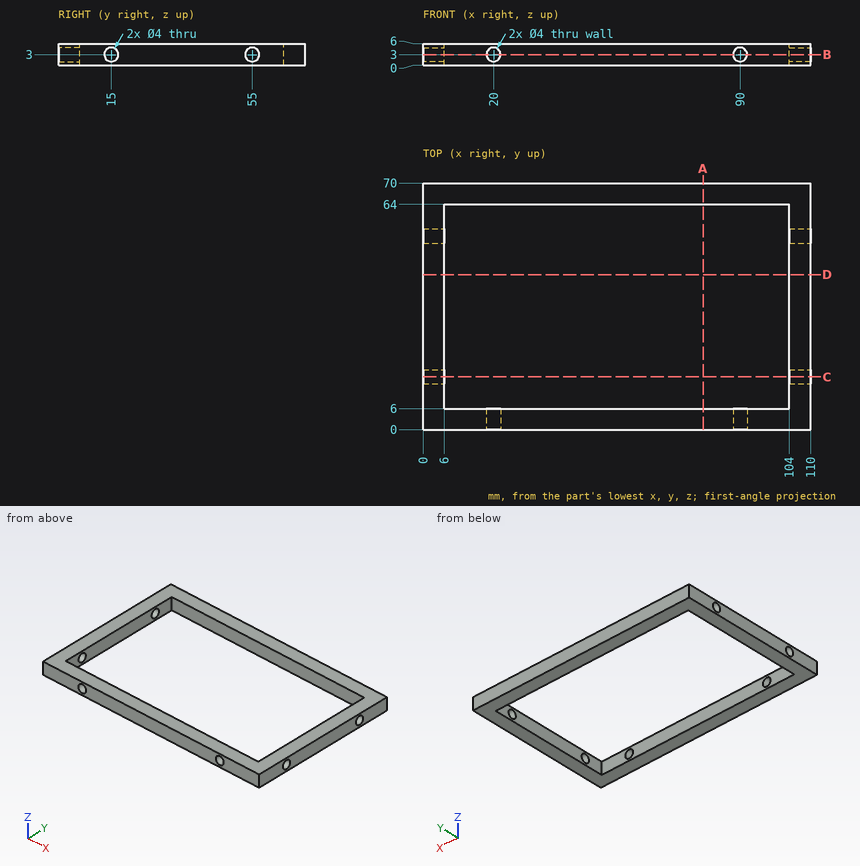
Geometry check sheet. Reference: drawing and pictorial views, mm from the part's lowest x, y, z. Round coordinates to 2 decimals unless told otherwise and drop trailing zeros. Write each loop counter-clockwise with the first axis right and the second up, starting at its lowest first coordinate (ties: lowest second). Pieces come first, ordered by that corner, then holes.
(1) Section check A-A (x = 79.5). Enter the section's corners in (y, z), plus the area to 3 significant figures.
Returned:
outline: (0, 0) - (6, 0) - (6, 6) - (0, 6) - close; (64, 0) - (70, 0) - (70, 6) - (64, 6) - close
area: 72.0 mm2
(2) Depth check by flat-ended pin: pin 1 Ø2.5 at (y, z) = (55, 3) entering from +X (3 decimals). Enter the tip coordinate at first touch or a pass-through.
Returned:
pin 1: passes through
(3) Section check D-D (y = 44). Enter the section's corners in (x, z).
Returned:
outline: (0, 0) - (6, 0) - (6, 6) - (0, 6) - close; (104, 0) - (110, 0) - (110, 6) - (104, 6) - close
(4) Section check C-C (y = 15). Enter the section's corners in (x, z), plus the area to 3 significant figures.
Returned:
outline: (0, 0) - (6, 0) - (6, 1) - (0, 1) - close; (0, 5) - (6, 5) - (6, 6) - (0, 6) - close; (104, 0) - (110, 0) - (110, 1) - (104, 1) - close; (104, 5) - (110, 5) - (110, 6) - (104, 6) - close
area: 24.0 mm2
(5) Material ranges on line 1 (X direction, y = 29, z = 4.5); line 2 (Y direction, x = 75, z = 3.35); line 3 (Z direction, x = 90, y = 1.8), recorded low to high.
Returned:
line 1: x = 0 to 6, 104 to 110
line 2: y = 0 to 6, 64 to 70
line 3: z = 0 to 1, 5 to 6
(6) Section check B-B (z = 3). Give the number of separate pieces and of enclosed holes in the cut face, plus the area to 3 significant figures.
Returned:
separate pieces: 6
enclosed holes: 0
area: 1,870 mm2
